Input: part model. Units: mm. Frame: model coordinates. A direction names the side the tool comes from. Give positions to 0.01 mm unless a question says otherwise; leave off trailing zeros. Loops run counter-clockwise (first coordinate to the right, second up) from the corner with the lowest first, then second, coordinate; pieces in that order, holes last. Notation, with made-up numbers: M -17,24.25 L 42,24.25 A23 ccw 42,48.25 Z; hole C 27.25,22 d7. An arc over 180 degrees is marked long. Use a Markdown table: item, result. Add a question column.
Autodesk Inventor part; units mm, degrees
ref_plane "YZ Plane" through (0, 0, 0) normal (1, 0, 0) x (0, 1, 0)
ref_plane "XZ Plane" through (0, 0, 0) normal (0, 1, 0) x (-1, 0, 0)
ref_plane "XY Plane" through (0, 0, 0) normal (0, 0, 1) x (1, 0, 0)
sketch "스케치1" plane through (0, 0, 0) normal (0, 0, 1) x (1, 0, 0)
  circle A0 centre (0, 0) radius 20
  dimension "d0" = 40
extrude "돌출1" add sketch "스케치1" along normal blind 70
sketch "스케치2" plane through (0, 0, 0) normal (0, 0, -1) x (-1, 0, 0)
  circle A0 centre (0, 0) radius 12.5
  dimension "d3" = 25
extrude "돌출2" cut sketch "스케치2" against normal blind 20
sketch "스케치3" plane through (0, 0, 20) normal (0, 0, -1) x (-1, 0, 0)
  circle A0 centre (0, 0) radius 15
  dimension "d6" = 30
extrude "돌출3" cut sketch "스케치3" against normal blind 20
sketch "스케치4" plane through (0, 0, 40) normal (0, 0, -1) x (-1, 0, 0)
  circle A0 centre (0, 0) radius 12.5
  dimension "d9" = 25
extrude "돌출4" cut sketch "스케치4" against normal up to next
properties part number "기본 투상 연습3"
1) Section query A-A, the plane x = 0. Return the cut outline in (y, z).
2) Pull-direction query (Z, two-part tool) for faces 3 (the cylindrical face through (14.985, 0.66, 29.86)), 4 (the flat face through (3.4, 12.3, 20)), 5 (the flat face through (9, 9, 70)), 6 (the cylindrical face through (-4.336, 19.524, 34.51)); classes: pulls with the +Z half, pulls with the -Z half, needs draft (parallel to the pull), parting line crosses it, or undercut.
3) Contact query for flat-ended pins moving along their axis: P1, Ø6, axis at x = 12.5, z = 56.5, coming from the +Y side; P2, Ø3, axis at x = -5.5, z = 45, coming from the -Y side; P3, Ø10, axis at y = 6.5, z = 52.5, coming from the -X side; P4, Ø18, axis at x = 0, y = 0, coming from the +Z side. Output: stop coordinate, or through.
4) Section query C-C, the plane z = 57. Return the cut outline in (x, y), and give its area (3 significant figures).
5) Ray query, line 1 (Y direction, x = 0, z = 63.5); line 2 (X direction, y = -0.5, z = 47.5); line 3 (X direction, y = 7, z = 20.5) (1 decimal). Return the intervals inside material, ascending. Write a range as [from, to].
6) Section query D-D, the plane y = 17. Return the cut outline in (x, z).
7) Reachability of faces 1 (the flat face through (3.4, 12.3, 40)), 2 (the flat face through (9, 9, 0)) from +Z, -Z, +X, -X, +Y, -Y: full face, straight path, thin tool, end or side. Return the list, or none.
Entries:
| question | item | result |
|---|---|---|
| 1 | outline | M -20,0 L -12.5,0 L -12.5,20 L -15,20 L -15,40 L -12.5,40 L -12.5,70 L -20,70 Z; M 12.5,0 L 20,0 L 20,70 L 12.5,70 L 12.5,40 L 15,40 L 15,20 L 12.5,20 Z |
| 2 | face 3 | undercut |
| 2 | face 4 | undercut |
| 2 | face 5 | pulls with the +Z half |
| 2 | face 6 | needs draft |
| 3 | P1 | stops at y = 17.6 |
| 3 | P2 | stops at y = -19.6 |
| 3 | P3 | stops at x = -19.94 |
| 3 | P4 | passes through |
| 4 | outline | C 0,0 d40; hole C 0,0 d25 |
| 4 | area | 766 mm² |
| 5 | line 1 | y = [-20, -12.5], [12.5, 20] |
| 5 | line 2 | x = [-19.99, -12.49], [12.49, 19.99] |
| 5 | line 3 | x = [-18.7, -13.3], [13.3, 18.7] |
| 6 | outline | M -10.54,0 L 10.54,0 L 10.54,70 L -10.54,70 Z |
| 7 | face 1 | none |
| 7 | face 2 | -Z, +X, -X, +Y, -Y |
